Read the model definition and answer for the solid it produces. Units are mm, in the model's axes. Give positions to 0.01 mm unless a question says otherwise; leave off trailing zeros. Loops run counter-clockwise (first coordinate to the right, second up) from the corner with the lowest first, then second, coordinate; pieces in that order, holes last.
(1) Find section B-B, the plane x = -8. Write down the section's boundary in (y, z) (3 decimals), then the cut area to 3 significant figures.
(2) Find section A-A, the plane z = 0. Write down the section's boundary in (x, y) (3 decimals).
(3) Find section D-D, the plane x = 17.5. Write down the section's boundary in (y, z) (3 decimals).
(4) Find section C-C, the plane y = 1.6. State how many separate pieces and enclosed holes the cut face has, then the cut area to 3 significant figures.
(5) Straight lines are drawn through the part: probe 1 along Z at (x, y) = (150, 2.45); probe 2 along X at (y, z) = (0.95, 9); probe 3 along X at (y, z) = (2.1, 17.5). For each, find the intervals that lie inside material, in ascending order.
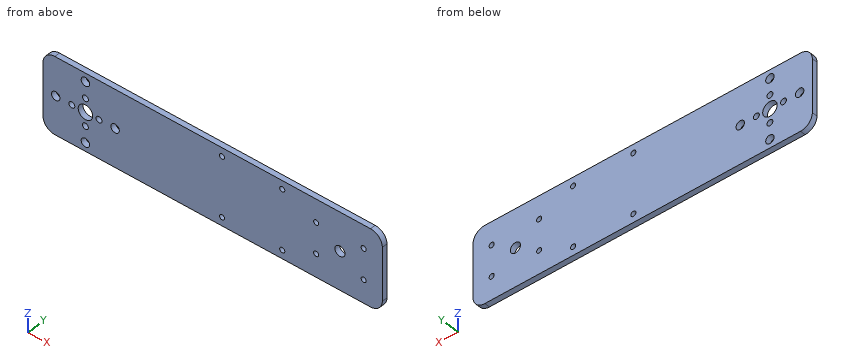
```python
from build123d import *

# Parameters (mm, degrees)
SKETCH1_W           = 200
SKETCH1_H           = 45
BOSS_EXTRUDE1_DEPTH = 3.175
SKETCH4_R           = 3
SKETCH4_R_2         = 1.5
CUT_EXTRUDE1_DEPTH  = 177.469064215
SKETCH5_R           = 4.25
CUT_EXTRUDE2_DEPTH  = 177.469064215
SKETCH10_R          = 1.5
CUT_EXTRUDE4_DEPTH  = 177.469064215
FILLET1_R           = 7
SKETCH11_R          = 2.5
CUT_EXTRUDE5_DEPTH  = 177.469064215
SKETCH12_R          = 1.75
CUT_EXTRUDE6_DEPTH  = 177.469064215


with BuildPart() as part:
    # Sketch1 → Boss-Extrude1 (new body)
    with BuildSketch(Plane(origin=(0, 0, 0), x_dir=(1, 0, 0), z_dir=(0, 1, 0))):
        with Locations((75, 0)):
            Rectangle(SKETCH1_W, SKETCH1_H)
    extrude(amount=BOSS_EXTRUDE1_DEPTH)

    # Sketch4 → Cut-Extrude1 (cut, through all)
    with BuildSketch(Plane(origin=(0, 3.175, 0), x_dir=(1, 0, 0), z_dir=(0, 1, 0))):
        with Locations(Location((150, 0, 0), (0, 0, 270))):
            Circle(SKETCH4_R)
        with Locations(Location((136, 9, 0), (0, 0, 270))):
            Circle(SKETCH4_R_2)
        with Locations(Location((164, 9, 0), (0, 0, 90))):
            Circle(SKETCH4_R_2)
        with Locations(Location((164, -9, 0), (0, 0, 270))):
            Circle(SKETCH4_R_2)
        with Locations(Location((136, -9, 0), (0, 0, 90))):
            Circle(SKETCH4_R_2)
    extrude(amount=-CUT_EXTRUDE1_DEPTH, mode=Mode.SUBTRACT)

    # Sketch5 → Cut-Extrude2 (cut, through all)
    with BuildSketch(Plane(origin=(0, 3.175, 0), x_dir=(1, 0, 0), z_dir=(0, 1, 0))):
        with Locations(Location((0, 0, 0), (0, 0, 270))):
            Circle(SKETCH5_R)
    extrude(amount=-CUT_EXTRUDE2_DEPTH, mode=Mode.SUBTRACT)

    # Sketch10 → Cut-Extrude4 (cut, through all)
    with BuildSketch(Plane(origin=(0, 3.175, 0), x_dir=(1, 0, 0), z_dir=(0, 1, 0))):
        with Locations(Location((80.5, -17.5, 0), (0, 0, 270))):
            Circle(SKETCH10_R)
        with Locations(Location((116, -17.5, 0), (0, 0, 270))):
            Circle(SKETCH10_R)
        with Locations(Location((116, 17.5, 0), (0, 0, 90))):
            Circle(SKETCH10_R)
        with Locations(Location((80.5, 17.5, 0), (0, 0, 90))):
            Circle(SKETCH10_R)
    extrude(amount=-CUT_EXTRUDE4_DEPTH, mode=Mode.SUBTRACT)

    # Fillet1
    fillet1_edges = [part.edges().sort_by_distance(p)[0] for p in [
        (-25, 1.5875, -22.5),
        (175, 1.5875, -22.5),
        (175, 1.5875, 22.5),
        (-25, 1.5875, 22.5),
    ]]
    fillet(fillet1_edges, radius=FILLET1_R)

    # Sketch11 → Cut-Extrude5 (cut, through all)
    with BuildSketch(Plane(origin=(0, 3.175, 0), x_dir=(1, 0, 0), z_dir=(0, 1, 0))):
        with Locations(Location((0, 17.5, 0), (0, 0, 270))):
            Circle(SKETCH11_R)
        with Locations(Location((17.5, 0, 0), (0, 0, 270))):
            Circle(SKETCH11_R)
        with Locations(Location((0, -17.5, 0), (0, 0, 270))):
            Circle(SKETCH11_R)
        with Locations(Location((-17.5, 0, 0), (0, 0, 270))):
            Circle(SKETCH11_R)
    extrude(amount=-CUT_EXTRUDE5_DEPTH, mode=Mode.SUBTRACT)

    # Sketch12 → Cut-Extrude6 (cut, through all)
    with BuildSketch(Plane(origin=(0, 3.175, 0), x_dir=(1, 0, 0), z_dir=(0, 1, 0))):
        with Locations(Location((0, 8, 0), (0, 0, 270))):
            Circle(SKETCH12_R)
        with Locations(Location((8, 0, 0), (0, 0, 270))):
            Circle(SKETCH12_R)
        with Locations(Location((0, -8, 0), (0, 0, 270))):
            Circle(SKETCH12_R)
        with Locations(Location((-8, 0, 0), (0, 0, 270))):
            Circle(SKETCH12_R)
    extrude(amount=-CUT_EXTRUDE6_DEPTH, mode=Mode.SUBTRACT)


solid = part.part
```
Entries:
1. outline: (0, -22.5) - (3.175, -22.5) - (3.175, -1.75) - (0, -1.75) - close; (0, 1.75) - (3.175, 1.75) - (3.175, 22.5) - (0, 22.5) - close
1. area: 132 mm2
2. outline: (-25, 0) - (-20, 0) - (-20, 3.175) - (-25, 3.175) - close; (-15, 0) - (-9.75, 0) - (-9.75, 3.175) - (-15, 3.175) - close; (-6.25, 0) - (-4.25, 0) - (-4.25, 3.175) - (-6.25, 3.175) - close; (4.25, 0) - (6.25, 0) - (6.25, 3.175) - (4.25, 3.175) - close; (9.75, 0) - (15, 0) - (15, 3.175) - (9.75, 3.175) - close; (20, 0) - (147, 0) - (147, 3.175) - (20, 3.175) - close; (153, 0) - (175, 0) - (175, 3.175) - (153, 3.175) - close
3. outline: (0, -22.5) - (3.175, -22.5) - (3.175, -2.5) - (0, -2.5) - close; (0, 2.5) - (3.175, 2.5) - (3.175, 22.5) - (0, 22.5) - close
4. separate pieces: 1
4. enclosed holes: 18
4. area: 8,700 mm2
5. probe 1: z = -22.5 to -3, 3 to 22.5
5. probe 2: x = -25 to -1.44, 1.44 to 134.5, 137.5 to 162.5, 165.5 to 175
5. probe 3: x = -24.71 to -2.5, 2.5 to 79, 82 to 114.5, 117.5 to 174.71
